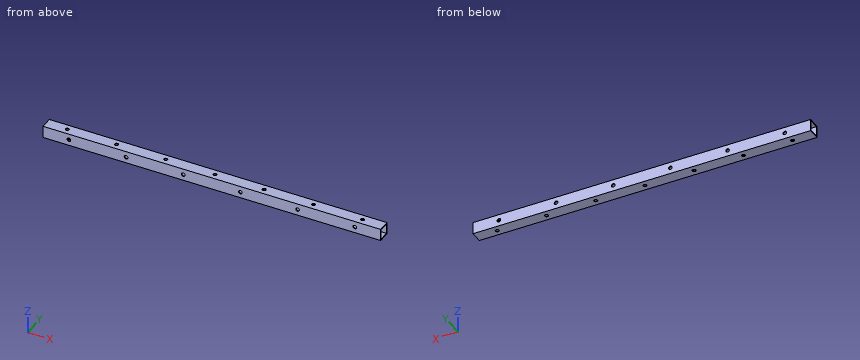
from build123d import *

# Parameters (mm, degrees)
SKETCH1_W               = 19.05
SKETCH1_H               = 19.05
SKETCH1_W_2             = 15.875
SKETCH1_H_2             = 15.875
TUBE_DEPTH              = 539.9532
SKETCH2_R               = 2.8956
REARWALLHOLES_DEPTH     = 541.373099178
LPATTERN1_COUNT         = 7
LPATTERN1_PITCH         = 78.74
SKETCH3_R               = 2.8956
REARTOPHOLEMASTER_DEPTH = 541.373099178
LPATTERN2_COUNT         = 6
LPATTERN2_PITCH         = 91.44


with BuildPart() as part:
    # Sketch1 → Tube (new body)
    with BuildSketch(Plane(origin=(0, 0, 0), x_dir=(0, -1, 0), z_dir=(1, 0, 0))):
        Rectangle(SKETCH1_W, SKETCH1_H)
        Rectangle(SKETCH1_W_2, SKETCH1_H_2, mode=Mode.SUBTRACT)
    extrude(amount=TUBE_DEPTH)

    # Sketch2 → RearWallHoles (cut, through all)
    with BuildSketch(Plane.XY.offset(9.525)):
        with Locations((506.1966, 0)):
            Circle(SKETCH2_R)
    rearwallholes = extrude(amount=-REARWALLHOLES_DEPTH, mode=Mode.SUBTRACT)

    # LPattern1: RearWallHoles ×7
    with Locations(*[(-i * LPATTERN1_PITCH, 0, 0) for i in range(1, LPATTERN1_COUNT)]):
        add(rearwallholes, mode=Mode.SUBTRACT)

    # Sketch3 → RearTopHoleMaster (cut, through all)
    with BuildSketch(Plane(origin=(0, 9.525, 0), x_dir=(1, 0, 0), z_dir=(0, 1, 0))):
        with Locations(Location((41.3766, 0, 0), (0, 0, 270))):
            Circle(SKETCH3_R)
    reartopholemaster = extrude(amount=-REARTOPHOLEMASTER_DEPTH, mode=Mode.SUBTRACT)

    # LPattern2: RearTopHoleMaster ×6
    with Locations(*[(i * LPATTERN2_PITCH, 0, 0) for i in range(1, LPATTERN2_COUNT)]):
        add(reartopholemaster, mode=Mode.SUBTRACT)


solid = part.part
Read the model definition and answer for the solid it produces. Units are mm, in the model's axes. Round coordinates to 2 decimals unless told otherwise and drop trailing zeros. Write each loop counter-clockwise with the first axis right and the second up, starting at its lowest first coordinate (ties: lowest second). Pieces come first, ordered by that corner, then holes. Notation, with made-up numbers: M 65,26.25 L 105,26.25 A20 ccw 105,37.25 Z; hole C 88.25,70.5 d1. An arc over 180 degrees is marked long. Use a Markdown table: item, result.
1) The part is cut by section A-A (x = 302.5). Write down the section's boundary in (y, z) (1 decimal), plus the area to 3 significant figures.
Answers follow:
| item | result |
|---|---|
| outline | M -9.5,-9.5 L 9.5,-9.5 L 9.5,9.5 L -9.5,9.5 Z; hole M -7.9,-7.9 L 7.9,-7.9 L 7.9,7.9 L -7.9,7.9 Z |
| area | 111 mm2 |
2) The part is cut by section B-B (z = 0). Give the number of separate pieces and of enclosed holes in the cut face, plus the area to 3 significant figures.
Answers follow:
| item | result |
|---|---|
| separate pieces | 14 |
| enclosed holes | 0 |
| area | 1,600 mm2 |
3) A flat-ended cylindrical pin translates along its axis: pin 1 (4 mm diameter, centred on y = 6.5, z = -7, fed in from +X). Find the tip coordinate at first contact, or state that the pin passes through.
Answers follow:
| item | result |
|---|---|
| pin 1 | stops at x = 539.95 |
4) Straight lines are drawn through the part: line 1 along Z through (x, y) = (448.5, 2.25) (1 decimal); line 2 along Y through (x, z) = (425.5, 8.25) (3 decimals). For each, find the intervals that lie inside material, in ascending order. Write a range as [from, to].
Answers follow:
| item | result |
|---|---|
| line 1 | z = [-9.5, -7.9], [7.9, 9.5] |
| line 2 | y = [-9.525, -2.135], [2.135, 9.525] |
